```python
from build123d import *

# Parameters (mm, degrees)
SKETCH2_W           = 40
SKETCH2_H           = 6
BOSS_EXTRUDE2_DEPTH = 299
SKETCH4_R           = 3
CUT_EXTRUDE2_DEPTH  = 42
CUT_EXTRUDE4_DEPTH  = 42


with BuildPart() as part:
    # Sketch2 → Boss-Extrude2 (new body)
    with BuildSketch(Plane.XY):
        Rectangle(SKETCH2_W, SKETCH2_H)
    extrude(amount=BOSS_EXTRUDE2_DEPTH)

    # Sketch4 → Cut-Extrude2 (cut, symmetric)
    with BuildSketch(Plane(origin=(0, 3, 0), x_dir=(1, 0, 0), z_dir=(0, 1, 0))):
        with Locations(Location((0, -59.5, 0), (0, 0, 270))):
            Circle(SKETCH4_R)
        with Locations(Location((0, -239.5, 0), (0, 0, 270))):
            Circle(SKETCH4_R)
    extrude(amount=CUT_EXTRUDE2_DEPTH, both=True, mode=Mode.SUBTRACT)

    # Sketch5 → Cut-Extrude4 (cut, symmetric)
    with BuildSketch(Plane(origin=(0, 3, 0), x_dir=(1, 0, 0), z_dir=(0, 1, 0))):
        Polygon((-3, -299), (3, -299), (3, -281.386427855), (5.311461506, -281.386427855), (5.311461506, -276.386427855), (3, -276.386427855), (3, -269), (-3, -269), (-3, -276.386427855), (-5.311461506, -276.386427855), (-5.311461506, -281.386427855), (-3, -281.386427855), align=None)
    cut_extrude4 = extrude(amount=CUT_EXTRUDE4_DEPTH, both=True, mode=Mode.SUBTRACT)

    # Mirror2: Cut-Extrude4 across plane
    add(cut_extrude4.mirror(Plane.XY.offset(149.5)), mode=Mode.SUBTRACT)


solid = part.part
```
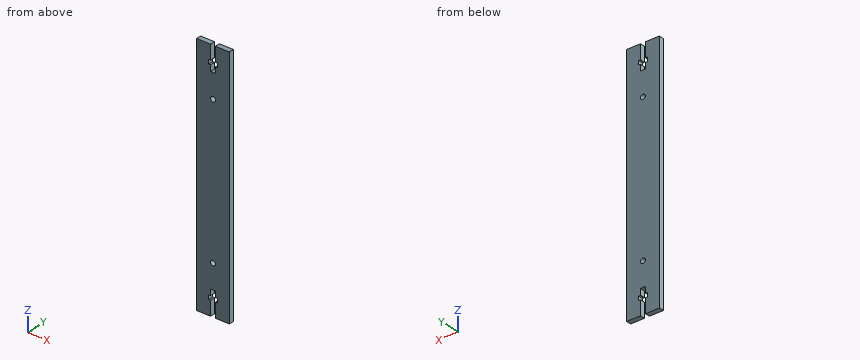
Geometry check sheet. Reference: the model listing, model coordinates, mm. Give positions to 0.01 mm unless a question says otherwise; leave off trailing zeros. Write each loop counter-clockwise with the first axis right and the second up, starting at its lowest first coordinate (ties: lowest second). Pieces come first, ordered by that corner, then holes. Notation, with made-up numbers: (-35, 46) -> (-18, 46) arc R33 ccw to (-18, 76) -> close; hole circle Ø1 at (27, -24). An arc over 180 degrees is marked (long way). Use one line per item in the form item = value.
Item 1: Sectioned sample at B-B on x = 0. Enter the section's corners in (y, z).
Results list:
outline = (-3, 30) -> (3, 30) -> (3, 56.5) -> (-3, 56.5) -> close; (-3, 62.5) -> (3, 62.5) -> (3, 236.5) -> (-3, 236.5) -> close; (-3, 242.5) -> (3, 242.5) -> (3, 269) -> (-3, 269) -> close
Item 2: Scan line: line 1 (X direction, y = 0.6, z = 59.5). Record every from-to range of solid material in increasing order.
Results list:
line_1 = -20 to -3, 3 to 20
Item 3: Sectioned sample at A-A on z = 239.5. Enter the section's corners in (x, y), plus the area to 3 significant figures.
Results list:
outline = (-20, -3) -> (-3, -3) -> (-3, 3) -> (-20, 3) -> close; (3, -3) -> (20, -3) -> (20, 3) -> (3, 3) -> close
area = 204 mm2
Item 4: Sectioned sample at C-C on y = -0.8. Count the separate pieces of the cut face and the enclosed holes in it, plus the area to 3 significant figures.
Results list:
separate_pieces = 1
enclosed_holes = 2
area = 11,500 mm2
Item 5: Depth check by flat-ended pin: pin 1 Ø5 at (x, z) = (0, 239.5) entering from +Y; pin 2 Ø3 at (x, y) = (0.5, 0.5) entering from -Z. Enter the tip coordinate at first touch or a pass-through.
Results list:
pin_1 = through
pin_2 = 30
